```python
from build123d import *

# Parameters (mm, degrees)
RESSALTO_EXTRUS_O2_DEPTH = 8
ESBO_O4_W                = 5.2
ESBO_O4_H                = 5.2
CORTE_EXTRUS_O1_DEPTH    = 4.5
CHANFRO1_SIZE            = 1
CHANFRO2_SIZE            = 1
FURO_ROSCADO_DE_M21_D    = 1.6


with BuildPart() as part:
    # Esboço2 → Ressalto-extrusão2 (new body)
    with BuildSketch(Plane(origin=(0, 0, 0), x_dir=(1, 0, 0), z_dir=(0, 1, 0))):
        with BuildLine():
            Line((-0.189366094, 0.757464375), (-2.189366094, 8.757464375))
            ThreePointArc((-2.189366094, 8.757464375), (-2.007429032, 9.615412209), (-1.219223594, 10))
            Line((-1.219223594, 10), (41.219223594, 10))
            ThreePointArc((41.219223594, 10), (42.007429032, 9.615412209), (42.189366094, 8.757464375))
            Line((42.189366094, 8.757464375), (40.189366094, 0.757464375))
            ThreePointArc((40.189366094, 0.757464375), (39.834635803, 0.211794562), (39.219223594, 0))
            Line((39.219223594, 0), (0.780776406, 0))
            ThreePointArc((0.780776406, 0), (0.165364197, 0.211794562), (-0.189366094, 0.757464375))
        make_face()
    extrude(amount=RESSALTO_EXTRUS_O2_DEPTH)

    # Esboço4 → Corte-extrusão1 (cut)
    with BuildSketch(Plane(origin=(0, 8, 0), x_dir=(1, 0, 0), z_dir=(0, 1, 0))):
        with Locations((28.5, 2.6)):
            Rectangle(ESBO_O4_W, ESBO_O4_H)
        with Locations((11.5, 2.6)):
            Rectangle(ESBO_O4_W, ESBO_O4_H)
    extrude(amount=-CORTE_EXTRUS_O1_DEPTH, mode=Mode.SUBTRACT)

    # Chanfro1
    chanfro1_edges = [part.edges().sort_by_distance(p)[0] for p in [
        (-2.007429032, 8, -9.615412209),
        (-1.189366094, 8, -4.757464375),
        (0.165364197, 8, -0.211794562),
        (4.840388203, 8, 0),
        (20, 8, 0),
        (35.159611797, 8, 0),
        (39.834635803, 8, -0.211794562),
        (41.189366094, 8, -4.757464375),
        (31.1, 8, -2.6),
        (28.5, 8, -5.2),
        (25.9, 8, -2.6),
        (8.9, 8, -2.6),
        (14.1, 8, -2.6),
        (11.5, 8, -5.2),
        (42.007429032, 8, -9.615412209),
        (20, 8, -10),
    ]]
    chamfer(chanfro1_edges, length=CHANFRO1_SIZE - 0.0001)  # a hair under: the kernel refuses the full size

    # Chanfro2
    chanfro2_edges = [part.edges().sort_by_distance(p)[0] for p in [
        (-1.189366094, 0, -4.757464375),
        (-2.007429032, 0, -9.615412209),
        (20, 0, -10),
        (42.007429032, 0, -9.615412209),
        (31.1, 5.25005, 0),
        (25.9, 5.25005, 0),
        (28.5, 3.5, 0),
        (8.9, 5.25005, 0),
        (14.1, 5.25005, 0),
        (11.5, 3.5, 0),
        (41.189366094, 0, -4.757464375),
        (39.834635803, 0, -0.211794562),
        (20, 0, 0),
        (0.165364197, 0, -0.211794562),
    ]]
    chamfer(chanfro2_edges, length=CHANFRO2_SIZE - 0.0001)  # a hair under: the kernel refuses the full size

    # Furo roscado de M21 (through all)
    with Locations(Plane(origin=(28.5, 3.5, -2.5), x_dir=(0, 0, 1), z_dir=(0, 1, 0))):
        with Locations((0, 0), (0, -17)):
            Hole(FURO_ROSCADO_DE_M21_D / 2)


solid = part.part
```
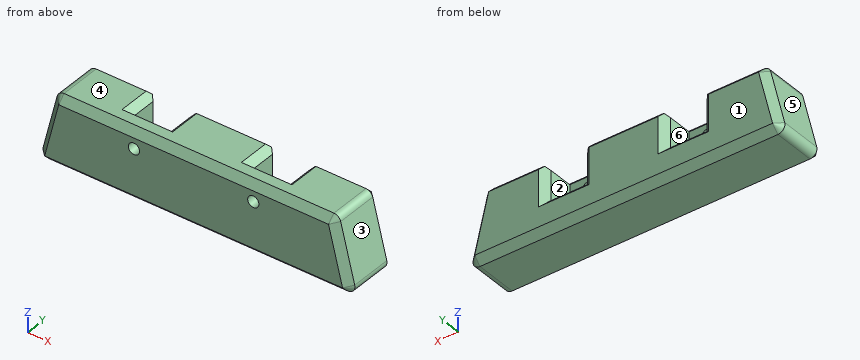
Verification items for the finished model (mm, model axes). Face numbers are marked on the shaded views. A direction names the side the tool comes from. Give positions to 0.01 mm unless a question says otherwise; leave off trailing zeros. Order: outer loops, then holes, each group sorted by start corner. A loop starts at its lowest first (then second) coordinate and runs counter-clockwise, first axis right, second up. Notation, with made-up numbers: M 13,18.25 L 45,18.25 A22 ccw 45,43.25 Z; hole C 2,-24.75 d6. An arc over 180 degrees is marked long. Answer in a Markdown table with one row per item. Add a question column.
Item 1: Section check C-C, the plane z = -2.5. Enter the section's corners in (x, y) (3 decimals), and give its area (3 significant figures).
Item 2: Gauge pin test, flat ends, axial feed: pin 1 (4 mm diameter, centred on y = 5.5, z = -2.5, fed in from -X) (3 decimals); pin 2 (4 mm diameter, centred on y = 6, z = -6.5, fed in from +X) (3 decimals); pin 3 (3 mm diameter, centred on y = 5, z = -2.5, fed in from +X). Record the tip position at first contact, or that the pin passes through.
Item 3: Section check B-B, the plane x = 11.5. Enter the section's corners in (y, z).
Item 4: Section check D-D, the plane x = 20. Enter the section's corners in (y, z).
Item 5: Tool access check on the marked faces 1 and 2. Record the directions out of +Z, -Z, +X, -X, +Y, -Y that give a thin tool (end or side, any length) a straight path to the whole face; none if there is none.
Item 6: Scan lines: probe 1 along X at (y, z) = (1.45, -2.5) (3 decimals); probe 2 along Z at (x, y) = (31, 6.5); probe 3 along X at (y, z) = (3, -0.25). Record each from-to range of solid material in increasing order. Write a range as from..to.
Item 7: Mould release check, pull along X, two halves, no side actions. Record for the marked faces 3, 4, 5 and 6: released by +X, released by -X, zero draft, split by the parting line, or undercut.
Item 8: Section check A-A, the plane y = 2. Enter the section's corners in (x, z).
Filled sheet:
| question | item | result |
|---|---|---|
| 1 | outline | M -0.625,1 L 0.406,0 L 10.7,0 L 10.7,3.5 L 8.9,3.5 L 8.9,7 L 7.9,8 L 0.406,8 L -0.625,7 Z; M 12.3,0 L 27.7,0 L 27.7,3.5 L 25.9,3.5 L 25.9,7 L 24.9,8 L 15.1,8 L 14.1,7 L 14.1,3.5 L 12.3,3.5 Z; M 29.3,0 L 39.594,0 L 40.625,1 L 40.625,7 L 39.594,8 L 32.1,8 L 31.1,7 L 31.1,3.5 L 29.3,3.5 Z |
| 1 | area | 268 mm^2 |
| 2 | pin 1 | stops at x = -1.125 |
| 2 | pin 2 | stops at x = 42.125 |
| 2 | pin 3 | stops at x = 41 |
| 3 | outline | M 0,-9 L 1,-10 L 7,-10 L 8,-9 L 8,-6.2 L 7,-5.2 L 3.5,-5.2 L 3.5,-3.3 L 0,-3.3 Z; M 0,-1.7 L 3.5,-1.7 L 3.5,-1 L 2.5,0 L 1,0 L 0,-1 Z |
| 4 | outline | M 0,-9 L 1,-10 L 7,-10 L 8,-9 L 8,-1 L 7,0 L 1,0 L 0,-1 Z |
| 5 | face 1 | +Z, -Z, +X, -X, +Y |
| 5 | face 2 | +Z, +Y |
| 6 | probe 1 | x = -0.625..10.7, 12.3..27.7, 29.3..40.625 |
| 6 | probe 2 | z = -10..-5.2 |
| 6 | probe 3 | x = 0.12..8.15, 14.85..25.15, 31.85..39.88 |
| 7 | face 3 | released by +X |
| 7 | face 4 | zero draft |
| 7 | face 5 | released by -X |
| 7 | face 6 | undercut |
| 8 | outline | M -2.19,-8.76 A1 ccw -1.22,-10 L 41.22,-10 A1 ccw 42.19,-8.76 L 40.19,-0.76 A1 ccw 39.22,0 L 0.78,0 A1 ccw -0.19,-0.76 Z; hole C 11.5,-2.5 d1.6; hole C 28.5,-2.5 d1.6 |
